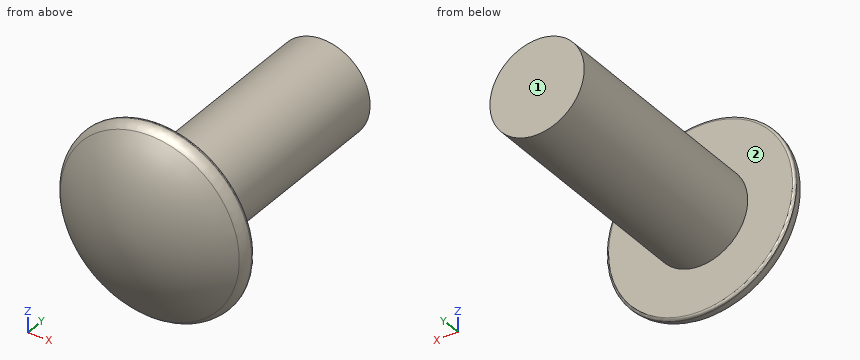
```python
from build123d import *

# Parameters (mm, degrees)
SKETCH2_W = 50
SKETCH2_H = 10
FILLET1_R = 3
FILLET2_R = 0.5


with BuildPart() as part:
    # Sketch2 → Revolve1 (revolve)
    with BuildSketch(Plane.YZ, mode=Mode.PRIVATE) as revolve1_sk:
        with BuildLine():
            Line((-10, 0), (-2, 0))
            Line((-2, 0), (-2, 20))
            ThreePointArc((-2, 20), (-7.925824036, 10.770329614), (-10, 0))
        make_face()
        Polygon((-2, 20), (-2, 0), (0, 0), (0, 10), (0, 20), align=None)
        with Locations((25, 5)):
            Rectangle(SKETCH2_W, SKETCH2_H)
    revolve(revolve1_sk.sketch.rotate(Axis((0, -34.621126621, 0), (0, 1, 0)), 180), axis=Axis((0, -34.621126621, 0), (0, 1, 0)))

    # Fillet1
    fillet1_edges = [part.edges().sort_by_distance(p)[0] for p in [
        (0, -2, 20),
    ]]
    fillet(fillet1_edges, radius=FILLET1_R)

    # Fillet2
    fillet2_edges = [part.edges().sort_by_distance(p)[0] for p in [
        (0, 0, 20),
    ]]
    fillet(fillet2_edges, radius=FILLET2_R)


solid = part.part
```
Check sheet for the modelled part. Datum: model origin and axes. Units: mm. Face numbers are marked on the shaded views. A direction names the side the tool comes from. Give positions to 0.01 mm unless a question says otherwise; leave off trailing zeros. Order: outer loops, then holes, each group sorted by start corner. A loop starts at its lowest first (then second) coordinate and runs counter-clockwise, first axis right, second up. Notation, with made-up numbers: (57, -8.75) -> (93, -8.75) arc R17 cw to (93, 19.25) -> close; hole circle Ø8 at (-21.75, 67). An arc over 180 degrees is marked (long way). Use CSV: the item, a comma, the result in double quotes. Start each with the question number.
1) Material ranges on line 1 (Y direction, x = 7, z = 9); line 2 (Y direction, x = 3.5, z = 18); line 3 (X direction, y = 45.5, z = -5), recorded low to high. Write a range as from..to.
2) Set-up check for the marked faces 1 and 2: record each of +Z, -Z, +X, -X, +Y, -Y from which the full face is reachable in a straight line by a thin tool's end or side.
3) Go/stop test with flat-tipped pins: P1, Ø5, axis at y = -2, z = -4, coming from the -X side; P2, Ø1, axis at y = -0.5, z = 8, coming from the -X side; P3, Ø12, axis at x = 1, y = 2.5, coming from the -Z side; P4, Ø1, axis at x = 9.5, y = 39, coming from the -Z side. Record where each tip stops, or that it passes through.
4) Sectioned sample at A-A, the plane y = 13.5. Record the boundary of the cut face in (x, z).
Recorded:
1,line 1,"-7.66..0"
1,line 2,"-3.47..0"
1,line 3,"-8.66..8.66"
2,face 1,"+Z, -Z, +X, -X, +Y"
2,face 2,"+Y"
3,P1,"x = -19.92"
3,P2,"x = -18.54"
3,P3,"z = -20"
3,P4,"z = -4.36"
4,outline,"circle Ø20 at (0, 0)"
